Model file for the job. Use its own axes, mm. A direction names the side the tool comes from. Give positions to 0.01 mm unless a question says otherwise; leave off trailing zeros. Loops run counter-clockwise (first coordinate to the right, second up) from the corner with the lowest first, then second, coordinate; pieces in that order, holes last. Notation, with made-up numbers: (67.5, -15) - (122.5, -15) arc R37 cw to (122.5, 23) - close; hole circle Ø6 at (82.25, -25). An arc over 180 degrees is marked (long way). Use a Markdown table: item, result.
from build123d import *

# Parameters (mm, degrees)
F4_T     = -2.54
F7_DEPTH = 2.54
F8_W     = 44.45
F8_H     = 114.3
F9_DEPTH = 25.4
F13_W    = 50.8
F13_H    = 127
F11_W    = 38.1
F11_H    = 88.9


with BuildPart() as f3:
    # F0 (on Top) → F3 section 0
    with BuildSketch(Plane.XY):
        with BuildLine():
            ThreePointArc((0, 79.1834323877), (-33.0563178037, -9.7165676123), (0, -98.6165676123))
            ThreePointArc((0, -98.6165676123), (33.0563178037, -9.7165676123), (0, 79.1834323877))
        make_face()
    # F2 (on offset) → F3 section 1
    with BuildSketch(Plane.XY.offset(38.1)):
        with BuildLine():
            ThreePointArc((0, 90.3536503496), (-42.4992821869, -11.2463496504), (0, -112.8463496504))
            ThreePointArc((0, -112.8463496504), (42.4992821869, -11.2463496504), (0, 90.3536503496))
        make_face()
    loft()

    # F4
    f4_openings = [f3.faces().sort_by_distance(p)[0] for p in [
        (0, -11.24635, 38.1),
    ]]
    offset(amount=F4_T, openings=f4_openings)

    # F6 (on offset) → F7 (join)
    with BuildSketch(Plane.XY.offset(35.56)):
        with BuildLine():
            ThreePointArc((0, 87.4059291422), (-40.4220024881, -10.8625479043), (0, -109.1310249507))
            ThreePointArc((0, -109.1310249507), (39.5185295328, -10.8625479043), (0, 87.4059291422))
        make_face()
    extrude(amount=-F7_DEPTH)

    # F8 (on offset) → F9 (join)
    with BuildSketch(Plane.XY.offset(35.56)):
        with Locations((0, -12.8250825944)):
            Rectangle(F8_W, F8_H)
    extrude(amount=F9_DEPTH)

    # F13 (on offset) → F14 section 0
    with BuildSketch(Plane.XY.offset(60.96)):
        with Locations((0, -12.9791411197)):
            Rectangle(F13_W, F13_H)
    # F11 (on offset) → F14 section 1
    with BuildSketch(Plane.XY.offset(76.2)):
        with Locations((0, -12.9365438215)):
            Rectangle(F11_W, F11_H)
    loft()


solid = f3.part
(1) Mould opens along Y. For faces 1 (the flat face through (0, -11, 2.54)), 2 (the flat face through (-1, -13, 76.2)) say: pulls with the +Y half, pulls with the -Y half, needs draft (parallel to the pull), parting line crosses it, or undercut.
Computed:
| item | result |
|---|---|
| face 1 | undercut |
| face 2 | needs draft |
(2) Pin check, flat tips, straight feed: P1, Ø1.5, axis at y = 4.5, z = 52, coming from the -X side (3 decimals); P2, Ø7.5, axis at y = -30.5, z = 54, coming from the +X side (3 decimals); P3, Ø1.5, axis at y = -58.5, z = 33, coming from the -X side. Stop position of each tip, or through.
Computed:
| item | result |
|---|---|
| P1 | x = -22.225 |
| P2 | x = 22.225 |
| P3 | x = -33.38 |
(3) Drill centre lines: probe 1 along Z at (x, y) = (0, -44); probe 2 along Y at (x, z) = (-8, 6); probe 3 along X at (y, z) = (3, 41.5) (3 decimals). Where is each one in solid material? Low to high. Write a range as [from, to].
Computed:
| item | result |
|---|---|
| probe 1 | [0, 2.54], [33.02, 76.2] |
| probe 2 | [-90.96, -86.45], [66.58, 71.05] |
| probe 3 | [-22.225, 22.225] |
(4) Slice it at A-A, the plane z = 59. Write the cut outline in (x, y) (3 decimals), plus the area to 3 significant figures.
Computed:
| item | result |
|---|---|
| outline | (-22.225, -69.975) - (22.225, -69.975) - (22.225, 44.325) - (-22.225, 44.325) - close |
| area | 5,080 mm² |
(5) 3-axis set-ups, long thin cutter, end or side, ignore diameter. For faces 3 (the flat face through (-1, -10, 33.02)), 4 (the flat face through (0, -11, 0)): which of +Z, -Z, +X, -X, +Y, -Y reach the whole face in a straight line?
Computed:
| item | result |
|---|---|
| face 3 | none |
| face 4 | -Z, +X, -X, +Y, -Y |
